The listing builds one solid part. Answer for the finished solid, in the listing's coordinates (mm). A direction names the side the tool comes from. Coordinates: 2 decimals unless noted, no trailing zeros. Loops run counter-clockwise (first coordinate to the right, second up) from the corner with the lowest first, then second, coordinate; pieces in that order, holes last. Notation, with made-up numbers: (35, 43.25) - (62, 43.25) arc R23 cw to (62, 59.25) - close; hole circle Ø5 at (27, -28.75). An arc over 180 degrees is marked (long way). Return JSON: item names as keys, results as strings. Group by question number.
1. Section A-A (x = 44.5) is taken. Write down the section's boundary in (y, z), and give its area (3 significant figures).
2. Which of the six approach directions +Z, -Z, +X, -X, +Y, -Y give full straight-line access (tool end or side, diameter ignored) to faces 4 (the face through (43, 2, 33)), 5 (the face through (-45.964, 2.507, -34.825)), 6 (the face through (-4, 2, 40))?
3. The mould has two halves that part along X. Classify faces 1 (the face through (-1, 0, -1)), 2 (the face through (-47.233, 0.986, -33.893)), 3 (the face through (-51.5, 1, 1)): pulls with the +X half, pulls with the -X half, needs draft (parallel to the pull), parting line crosses it, or undercut.
4. Find the intervals of material crossed by line 1 along X through (y, z) = (1.75, 34.5); line 2 along X through (y, z) = (2.45, -34.5); line 3 along X through (y, z) = (2.6, 11.5), in increasing order.
5. Each of these flat-tipped pins is pushed along its axis until it touches: P1, Ø4, axis at x = -44.5, z = 34.5, coming from the -Y side; P2, Ø0.8, axis at x = 5, y = 2.5, coming from the -Z side; P3, Ø1.7, axis at x = 45, z = 34.5, coming from the -Y side. Where does it stop, or does it pass through?
6. Section D-D (z = 6) is taken. Write down the section's boundary in (x, y).
7. Section B-B (z = 34.5) is taken. Write down the section's boundary in (x, y).
8. Section C-C (x = 8) is taken. Write down the section's boundary in (y, z).
```python
from build123d import *

# Parameters (mm, degrees)
SKETCH1_W           = 103
SKETCH1_H           = 83
BOSS_EXTRUDE1_DEPTH = 2
SKETCH2_W           = 96.5
SKETCH2_H           = 76.5
BOSS_EXTRUDE2_DEPTH = 1
CHAMFER1_SIZE       = 1
SKETCH3_R           = 1.5
CUT_EXTRUDE1_DEPTH  = 67.208005558
SKETCH5_R           = 2.8
CUT_EXTRUDE2_DEPTH  = 2


with BuildPart() as part:
    # Sketch1 → Boss-Extrude1 (new body)
    with BuildSketch(Plane(origin=(0, 0, 0), x_dir=(1, 0, 0), z_dir=(0, 1, 0))):
        Rectangle(SKETCH1_W, SKETCH1_H)
    extrude(amount=BOSS_EXTRUDE1_DEPTH)

    # Sketch2 → Boss-Extrude2 (add)
    with BuildSketch(Plane(origin=(0, 2, 0), x_dir=(1, 0, 0), z_dir=(0, 1, 0))):
        Rectangle(SKETCH2_W, SKETCH2_H)
    extrude(amount=BOSS_EXTRUDE2_DEPTH)

    # Chamfer1
    chamfer1_edges = [part.edges().sort_by_distance(p)[0] for p in [
        (51.5, 1, 41.5),
        (-51.5, 1, 41.5),
        (-51.5, 1, -41.5),
        (51.5, 1, -41.5),
    ]]
    chamfer(chamfer1_edges, length=CHAMFER1_SIZE)

    # Sketch3 → Cut-Extrude1 (cut, through all)
    with BuildSketch(Plane(origin=(0, 3, 0), x_dir=(1, 0, 0), z_dir=(0, 1, 0))):
        with Locations(Location((-44.5, 34.5, 0), (0, 0, 270))):
            Circle(SKETCH3_R)
        with Locations(Location((44.5, 34.5, 0), (0, 0, 270))):
            Circle(SKETCH3_R)
        with Locations(Location((44.5, -34.5, 0), (0, 0, 270))):
            Circle(SKETCH3_R)
        with Locations(Location((-44.5, -34.5, 0), (0, 0, 270))):
            Circle(SKETCH3_R)
    extrude(amount=-CUT_EXTRUDE1_DEPTH, mode=Mode.SUBTRACT)

    # Sketch5 → Cut-Extrude2 (cut)
    with BuildSketch(Plane.XZ):
        with Locations(Location((-44.5, 34.5, 0), (0, 0, 270))):
            Circle(SKETCH5_R)
        with Locations(Location((44.5, 34.5, 0), (0, 0, 270))):
            Circle(SKETCH5_R)
        with Locations(Location((44.5, -34.5, 0), (0, 0, 270))):
            Circle(SKETCH5_R)
        with Locations(Location((-44.5, -34.5, 0), (0, 0, 270))):
            Circle(SKETCH5_R)
    extrude(amount=-CUT_EXTRUDE2_DEPTH, mode=Mode.SUBTRACT)


solid = part.part
```
The answers:
{
 "1": {"outline": "(0, -41.5) - (2, -41.5) - (2, -38.25) - (3, -38.25) - (3, -36) - (2, -36) - (2, -37.3) - (0, -37.3) - close; (0, -31.7) - (2, -31.7) - (2, -33) - (3, -33) - (3, 33) - (2, 33) - (2, 31.7) - (0, 31.7) - close; (0, 37.3) - (2, 37.3) - (2, 36) - (3, 36) - (3, 38.25) - (2, 38.25) - (2, 41.5) - (0, 41.5) - close", "area": "214 mm2"},
 "2": {"face 4": "-Y", "face 5": "+Y, -Y", "face 6": "+Y"},
 "3": {"face 1": "needs draft", "face 2": "undercut", "face 3": "pulls with the -X half"},
 "4": {"line 1": "x = -51.5 to -47.3, -41.7 to 41.7, 47.3 to 51.5", "line 2": "x = -48.25 to -46, -43 to 43, 46 to 48.25", "line 3": "x = -48.25 to 48.25"},
 "5": {"P1": "stops at y = 2", "P2": "stops at z = -38.25", "P3": "passes through"},
 "6": {"outline": "(-51.5, 0) - (51.5, 0) - (51.5, 2) - (48.25, 2) - (48.25, 3) - (-48.25, 3) - (-48.25, 2) - (-51.5, 2) - close"},
 "7": {"outline": "(-51.5, 0) - (-47.3, 0) - (-47.3, 2) - (-46, 2) - (-46, 3) - (-48.25, 3) - (-48.25, 2) - (-51.5, 2) - close; (-43, 2) - (-41.7, 2) - (-41.7, 0) - (41.7, 0) - (41.7, 2) - (43, 2) - (43, 3) - (-43, 3) - close; (46, 2) - (47.3, 2) - (47.3, 0) - (51.5, 0) - (51.5, 2) - (48.25, 2) - (48.25, 3) - (46, 3) - close"},
 "8": {"outline": "(0, -41.5) - (2, -41.5) - (2, -38.25) - (3, -38.25) - (3, 38.25) - (2, 38.25) - (2, 41.5) - (0, 41.5) - close"}
}
